Autodesk Inventor part; units mm, degrees
ref_plane "YZ Plane" through (0, 0, 0) normal (1, 0, 0) x (0, 1, 0)
ref_plane "XZ Plane" through (0, 0, 0) normal (0, 1, 0) x (-1, 0, 0)
ref_plane "XY Plane" through (0, 0, 0) normal (0, 0, 1) x (1, 0, 0)
sketch "Sketch1" plane through (0, 0, 0) normal (0, 1, 0) x (-1, 0, 0)
  circle A0 centre (0, 0) radius 4.5
  line L0 (0, 0) -> (0, -15)
  circle A1 centre (0, -15) radius 0.5
  circle A2 centre (0, -15) radius 1.5
  line L1 (4.3151, -1.2768) -> (1.4994, -15.0417)
  line L2 (-4.3151, -1.2768) -> (-1.4994, -15.0417)
  circle A3 centre (0, -6) radius 0.5
  circle A4 centre (0, -9) radius 0.5
  circle A5 centre (0, -12) radius 0.5
  line L3 (0, 0) -> (-1.4994, 0)
  circle A6 centre (0, 15) radius 0.5
  circle A7 centre (0, 15) radius 1.5
  line L4 (4.3151, 1.2768) -> (1.4994, 15.0417)
  line L5 (-4.3151, 1.2768) -> (-1.4994, 15.0417)
  circle A8 centre (0, 6) radius 0.5
  circle A9 centre (0, 9) radius 0.5
  circle A10 centre (0, 12) radius 0.5
  circle A11 centre (0, 0) radius 2.5
  dimension "d0" = 9
  dimension "d3" = 3
  dimension "d1" = 15
  dimension "d2" = 1
  dimension "d4" = 1
  dimension "d5" = 1
  dimension "d6" = 1
  dimension "d8" = 3
  dimension "d9" = 3
  dimension "d10" = 3
  dimension "d13" = 5
extrude "Extrusion1" add sketch "Sketch1" along normal blind 2.5 contours A0 L5 A7 L4 | L1 A2 L0 A5 A4 A3 A0 | A7 | L0 A3 A4 A5 A2 L2 A0 | A2
extrude "Extrusion2" add sketch "Sketch1" along normal blind 5.5 contours A0
properties part number "180Horn"
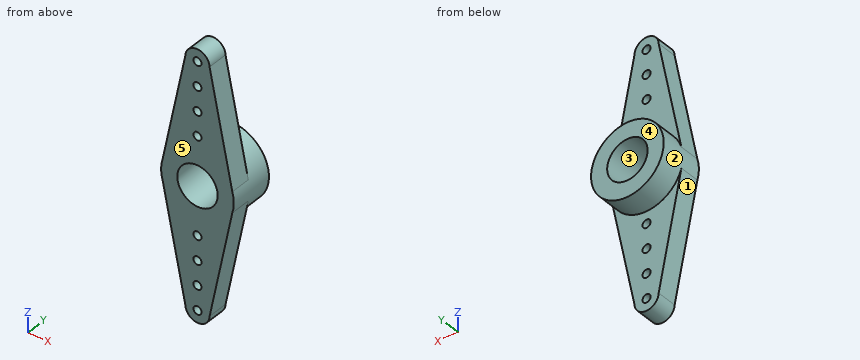
Design review of the part built by this model. Coordinates are the model's own, in mm. Face numbers are marked on the shaded views. A direction names the side the tool comes from. Coordinates: 2 decimals unless noted, no trailing zeros. Order: outer loops, then holes, each group sorted by start corner. A loop starts at its lowest first (then second) coordinate and runs counter-clockwise, first axis right, second up. Notation, with made-up numbers: (51, -36.75) -> (64, -36.75) arc R14 ccw to (64, -13.75) -> close; hole circle Ø2 at (-7, 56.25). An arc over 180 degrees is marked (long way). One line per item, written item: value. Start each with the question number.
Q1. Tool access review of the marked faces 1 and 2: name each direction out of +Z, -Z, +X, -X, +Y, -Y from which nothing blocks a thin tool from reaching the whole face with its end or side.
Q2. Take a section at C-C, the plane y = 4.35. State the section outline as (x, z) points.
Q3. Take a section at B-B, the plane y = 0.85. Give the number of separate pieces and of enclosed holes in the cut face, then the cut area to 3 significant figures.
Q4. Take a section at A-A, the plane z = 0. State the section outline as (x, y) points.
Q5. Mouldability with a two-part tool opening along Y and no side actions: class the marked faces 3, 4 and 5 as pulls with the +Y half, pulls with the -Y half, needs draft (parallel to the pull), parting line crosses it, or undercut.
Q6. Insertion check: pin 1 Ø2.5 at (x, z) = (-1, 10.5) entering from +Y; pin 2 Ø1 at (x, y) = (1, 1) entering from -Z. Each pin has a flat end and moves straight along its axis. Give the tip position at first contact, or say it passes through.
Q7. For probe 1 along Z at (x, y) = (-0.75, 5.1); probe 2 along X at (y, z) = (3, 1.5); probe 3 along X at (y, z) = (3, 0.5), list the stretches that pass through material, from the lowest coordinate up.
Values follow:
1. face 1: -Z, -X, +Y, -Y
1. face 2: +Y
2. outline: circle Ø9 at (0, 0); hole circle Ø5 at (0, 0)
3. separate pieces: 1
3. enclosed holes: 9
3. area: 164 mm2
4. outline: (-4.5, 0) -> (-2.5, 0) -> (-2.5, 5.5) -> (-4.5, 5.5) -> close; (2.5, 0) -> (4.5, 0) -> (4.5, 5.5) -> (2.5, 5.5) -> close
5. face 3: needs draft
5. face 4: pulls with the +Y half
5. face 5: pulls with the -Y half
6. pin 1: stops at y = 2.5
6. pin 2: stops at z = -16.41
7. probe 1: z = -4.44 to -2.38, 2.38 to 4.44
7. probe 2: x = -4.24 to -2, 2 to 4.24
7. probe 3: x = -4.47 to -2.45, 2.45 to 4.47
